```python
from build123d import *

# Parameters (mm, degrees)
SKETCH_1_R      = 60
SKETCH_1_R_2    = 2.6
SKETCH_1_R_3    = 2.1
EXTRUDE_1_DEPTH = 5
FILLET_1_R      = 8


with BuildPart() as part:
    # 草图1 → 凸台-拉伸1 (new body)
    with BuildSketch(Plane(origin=(0, 0, 0), x_dir=(1, 0, 0), z_dir=(0, 1, 0))):
        with Locations(Location((0, 0, 0), (0, 0, 270))):
            Circle(SKETCH_1_R)
        with Locations(Location((0, 53.5, 0), (0, 0, 270))):
            Circle(SKETCH_1_R_2, mode=Mode.SUBTRACT)
        with Locations(Location((53.5, 0, 0), (0, 0, 90))):
            Circle(SKETCH_1_R_2, mode=Mode.SUBTRACT)
        with Locations(Location((0, -53.5, 0), (0, 0, 90))):
            Circle(SKETCH_1_R_2, mode=Mode.SUBTRACT)
        with Locations(Location((-53.5, 0, 0), (0, 0, 270))):
            Circle(SKETCH_1_R_2, mode=Mode.SUBTRACT)
        with Locations(Location((-1.944543648, 19.268659787, 0), (0, 0, 270))):
            Circle(SKETCH_1_R_3, mode=Mode.SUBTRACT)
        with Locations(Location((19.268659787, -1.944543648, 0), (0, 0, 90))):
            Circle(SKETCH_1_R_3, mode=Mode.SUBTRACT)
        with Locations(Location((1.944543648, -19.268659787, 0), (0, 0, 270))):
            Circle(SKETCH_1_R_3, mode=Mode.SUBTRACT)
        with Locations(Location((-19.268659787, 1.944543648, 0), (0, 0, 90))):
            Circle(SKETCH_1_R_3, mode=Mode.SUBTRACT)
        Polygon((-5.656854249, 36.769552622), (36.769552622, -5.656854249), (48.083261121, 5.656854249), (5.656854249, 48.083261121), align=None, mode=Mode.SUBTRACT)
    extrude(amount=EXTRUDE_1_DEPTH)

    # 圆角1
    fillet_1_edges = [part.edges().sort_by_distance(p)[0] for p in [
        (36.769552622, 2.5, 5.656854249),
        (48.083261121, 2.5, -5.656854249),
        (5.656854249, 2.5, -48.083261121),
        (-5.656854249, 2.5, -36.769552622),
    ]]
    fillet(fillet_1_edges, radius=FILLET_1_R - 0.0001)  # a hair under: the kernel refuses the full size


solid = part.part
```
Build history of the part. All positions in model axes, mm. A direction names the side the tool comes from. Give positions to 0.01 mm unless a question says otherwise; leave off trailing zeros. Loops run counter-clockwise (first coordinate to the right, second up) from the corner with the lowest first, then second, coordinate; pieces in that order, holes last. Notation, with made-up numbers: (36.5, 46.5) -> (70.5, 46.5) arc R28 ccw to (70.5, 72.5) -> close; hole circle Ø4 at (23, 79). An arc over 180 degrees is marked (long way). One line per question, with ' | ' between items.
Q1. Cut at A-A, the plane x = 53.5. Write the cut outline in (y, z).
Filled sheet:
outline: (0, -27.16) -> (5, -27.16) -> (5, -2.6) -> (0, -2.6) -> close; (0, 2.6) -> (5, 2.6) -> (5, 27.16) -> (0, 27.16) -> close
Q2. Cut at B-B, the plane y = 2.85. Count the separate pieces of the cut face and the enclosed holes in it, plus the area to 3 significant figures.
Filled sheet:
separate pieces: 1 | enclosed holes: 9 | area: 10,300 mm²
Q3. Drop flat-ended pins along their axis: pin 1 (1.5 mm diameter, centred on x = -31, y = 1.5, fed in from +Z); pin 2 (2 mm diameter, centred on x = -40, y = 1.5, fed in from +Z); pin 3 (2 mm diameter, centred on x = -38.5, y = 0.5, fed in from +Z). Give the stop position or say it passes through.
Filled sheet:
pin 1: stops at z = 51.82 | pin 2: stops at z = 45.6 | pin 3: stops at z = 46.84
Q4. Cut at D-D, the plane z = 47. Write the cut outline in (x, y), plus the area to 3 significant figures.
Filled sheet:
outline: (-37.3, 0) -> (37.3, 0) -> (37.3, 5) -> (-37.3, 5) -> close | area: 373 mm²
Q5. Drill centre lines: line 1 along X through (y, z) = (0.85, -3.5); line 2 along X through (y, z) = (4.75, -2); line 3 along Z through (x, y) = (53.5, 2.6). Where is each one in solid material? Low to high. Write a range as [from, to].
Filled sheet:
line 1: x = [-59.9, -20.68], [-17.86, 27.61], [44.47, 59.9] | line 2: x = [-59.97, -55.16], [-51.84, -21.37], [-17.17, 29.11], [43.88, 51.84], [55.16, 59.97] | line 3: z = [-27.16, -2.6], [2.6, 27.16]
Q6. Pull direction X, two halves, no side cores. Call faces 1 (the cylindrical face through (2.64, 2.46, -59.94)), 2 (the cylindrical face through (-2.343, 2.535, -36.682)), 3 (the flat face through (1, 0, -1)): pulls with the +X half, pulls with the -X half, needs draft (parallel to the pull), parting line crosses it, or undercut.
Filled sheet:
face 1: parting line crosses it | face 2: undercut | face 3: needs draft
Q7. Cut at C-C, the plane z = -33.5. Write the cut outline in (x, y).
Filled sheet:
outline: (-49.78, 0) -> (-1.64, 0) -> (-1.64, 5) -> (-49.78, 5) -> close; (20.24, 0) -> (49.78, 0) -> (49.78, 5) -> (20.24, 5) -> close
Q8. Tool access for faces 4 (the cylindrical face through (36.682, 2.535, 2.343)), 5 (the flat face through (1, 5, -1)): list every direction of +Z, -Z, +X, -X, +Y, -Y with a clear straight run to the whole face (end or side of a thin tool).
Filled sheet:
face 4: +Y, -Y | face 5: +Z, -Z, +X, -X, +Y
